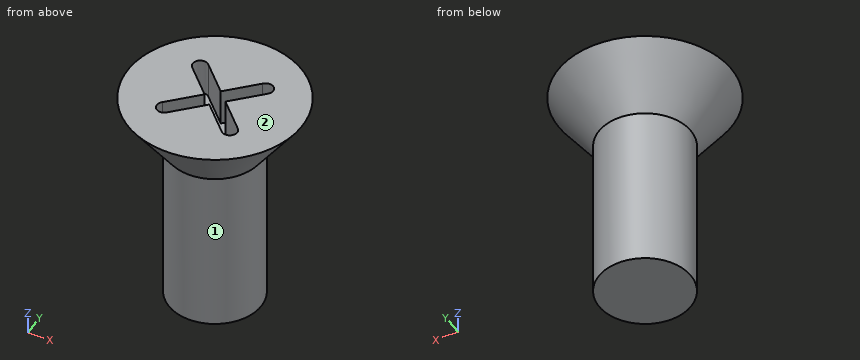
from build123d import *

# Parameters (mm, degrees)
POCKET_DEPTH = 1


with BuildPart() as part:
    # Sketch → Revolution (revolve)
    with BuildSketch(Plane.XZ):
        Polygon((0, 6), (-2.35, 6), (-1.25, 4.5), (-1.25, 0), (0, 0), align=None)
    revolve(axis=Axis((0, 0, 0), (0, 0, 1)))

    # Sketch001 (on Face1 of Revolution) → Pocket (cut)
    with BuildSketch(Plane(origin=(0, 0, 6), x_dir=(-1, 0, 0), z_dir=(0, 0, 1))):
        with BuildLine():
            Line((-0.74321, 1.028714), (0, 0.285504))
            Line((0.74321, 1.028714), (0, 0.285504))
            ThreePointArc((1.028714, 0.74321), (1.040084, 1.040084), (0.74321, 1.028714))
            Line((1.028714, 0.74321), (0.285504, 0))
            Line((1.028714, -0.74321), (0.285504, 0))
            ThreePointArc((0.74321, -1.028714), (1.040084, -1.040084), (1.028714, -0.74321))
            Line((0.74321, -1.028714), (0, -0.285504))
            Line((-0.74321, -1.028714), (0, -0.285504))
            ThreePointArc((-1.028714, -0.74321), (-1.040084, -1.040084), (-0.74321, -1.028714))
            Line((-1.028714, -0.74321), (-0.285504, 0))
            Line((-1.028714, 0.74321), (-0.285504, 0))
            ThreePointArc((-0.74321, 1.028714), (-1.040084, 1.040084), (-1.028714, 0.74321))
        make_face()
    extrude(amount=-POCKET_DEPTH, mode=Mode.SUBTRACT)


solid = part.part
Work out the finished part from the listing and answer in its coordinate system (mm). Face numbers are marked on the shaded views. A direction names the side the tool comes from. Coordinates: 2 decimals unless noted, no trailing zeros. Write each loop counter-clockwise with the first axis right and the second up, starting at its lowest first coordinate (ties: lowest second). Pieces come first, ordered by that corner, then holes. Notation, with made-up numbers: M 39,45.5 L 81,45.5 A32 cw 81,79.5 Z; hole C 56.25,-19.5 d2. An arc over 180 degrees is marked long. Use one line per item in the form item = value. Start each with the question number.
1. The part is cut by section B-B (z = 0.95). Give the vertices of the cut face in (x, y).
2. A tool of negligible diameter and unlimited length cuts with its end or side. For the marked faces 1 and 2, from which of +Z, -Z, +X, -X, +Y, -Y can it reach the whole face along a straight path? Write none if from no direction.
3. Each of these flat-tipped pins is pushed along its axis until it touches: P1, Ø2, axis at x = -1.5, z = 2.5, coming from the +Y side; P2, Ø1.5, axis at y = -1, z = 2, coming from the -X side; P3, Ø1, axis at x = 0, z = 2, coming from the +Y side. Where does it stop, or does it pass through?
4. Straight lines are drawn through the part: probe 1 along Z at (x, y) = (0.4, -0.5); probe 2 along X at (y, z) = (1.45, 5.5); probe 3 along Z at (x, y) = (-1.65, -0.55). For each, find the intervals that lie inside material, in ascending order. Write a range as from..to.
5. The part is cut by section A-A (z = 5.65). Give the vertices of the cut face in (x, y).
Evaluation:
q1.outline = C 0,0 d2.5
q2.face_1 = -Z
q2.face_2 = +Z, +X, -X, +Y, -Y
q3.P1 = 1.15
q3.P2 = -1.22
q3.P3 = 1.25
q4.probe_1 = 0..5
q4.probe_2 = -1.35..1.35
q4.probe_3 = 5.17..6
q5.outline = C 0,0 d4.19; hole M -1.03,-0.74 A0.2 ccw long -0.74,-1.03 L 0,-0.29 L 0.74,-1.03 A0.2 ccw long 1.03,-0.74 L 0.29,0 L 1.03,0.74 A0.2 ccw long 0.74,1.03 L 0,0.29 L -0.74,1.03 A0.2 ccw long -1.03,0.74 L -0.29,0 Z
